from build123d import *

# Parameters (mm, degrees)
EYELID_OUTLINE_R   = 1.25
EYELID_DEPTH       = 3
SKETCH1_R          = 1.5
SKETCH1_W          = 68
SKETCH1_H          = 13
CUT_EXTRUDE1_DEPTH = 48.130138977


# Read off the part's stored shape, not the designer's step: eyelid
with BuildPart() as part:
    # eyelid outline → eyelid (new body)
    with BuildSketch(Plane(origin=(0, 0, 0), x_dir=(1, 0, 0), z_dir=(0, 1, 0))):
        with BuildLine():
            Line((28, -2), (28, -3.803847577))
            ThreePointArc((28, -3.803847577), (27.598076211, -5.303847577), (26.5, -6.401923789))
            ThreePointArc((26.5, -6.401923789), (25.102222521, -9.776457136), (28, -12))
            Line((28, -12), (29.1, -12))
            Line((29.1, -12), (29.1, -16))
            Line((29.1, -16), (30.9, -25))
            Line((30.9, -25), (32.4, -25))
            Line((32.4, -25), (33.9, -23.5))
            Line((33.9, -23.5), (33.9, -22.5))
            Line((33.9, -22.5), (33.4, -22))
            Line((33.4, -22), (32.9, -21))
            Line((32.9, -21), (32.9, -12))
            Line((32.9, -12), (34, -12))
            Line((34, -12), (34, -1.200719678))
            Line((34, -1.200719678), (31.366635055, 8.507890769))
            ThreePointArc((31.366635055, 8.507890769), (0, 32.5), (-31.366635055, 8.507890769))
            Line((-31.366635055, 8.507890769), (-34, -1.200719678))
            Line((-34, -1.200719678), (-34, -12))
            Line((-34, -12), (-32.9, -12))
            Line((-32.9, -12), (-32.9, -21))
            Line((-32.9, -21), (-33.4, -22))
            Line((-33.4, -22), (-33.9, -22.5))
            Line((-33.9, -22.5), (-33.9, -23.5))
            Line((-33.9, -23.5), (-32.4, -25))
            Line((-32.4, -25), (-30.9, -25))
            Line((-30.9, -25), (-29.1, -16))
            Line((-29.1, -16), (-29.1, -12))
            Line((-29.1, -12), (-28, -12))
            ThreePointArc((-28, -12), (-25.102222521, -9.776457136), (-26.5, -6.401923789))
            ThreePointArc((-26.5, -6.401923789), (-27.598076211, -5.303847577), (-28, -3.803847577))
            Line((-28, -3.803847577), (-28, -2))
            Line((-28, -2), (-25.57587166, 6.937203242))
            ThreePointArc((-25.57587166, 6.937203242), (0, 26.5), (25.57587166, 6.937203242))
            Line((25.57587166, 6.937203242), (28, -2))
        make_face()
        with Locations((-28, -9)):
            Circle(EYELID_OUTLINE_R, mode=Mode.SUBTRACT)
        with Locations((28, -9)):
            Circle(EYELID_OUTLINE_R, mode=Mode.SUBTRACT)
    extrude(amount=EYELID_DEPTH)

    # Sketch1 → Cut-Extrude1 (cut, through all)
    with BuildSketch(Plane(origin=(0, 0, 0), x_dir=(1, 0, 0), z_dir=(0, 1, 0))):
        with Locations(Location((-28, -9, 0), (0, 0, 270))):
            Circle(SKETCH1_R)
        with Locations(Location((28, -9, 0), (0, 0, 270))):
            Circle(SKETCH1_R)
        with Locations((0, -18.5)):
            Rectangle(SKETCH1_W, SKETCH1_H)
    extrude(amount=CUT_EXTRUDE1_DEPTH, mode=Mode.SUBTRACT)


solid = part.part
Can you work these out from the model? Positions are in its coordinate system, mm. A direction names the side the tool comes from. Round coordinates to 2 decimals unless told otherwise and drop trailing zeros. Loops run counter-clockwise (first coordinate to the right, second up) from the corner with the lowest first, then second, coordinate; pieces in that order, holes last. Notation, with made-up numbers: (82.5, 43) - (117.5, 43) arc R22 cw to (117.5, 72) - close; hole circle Ø11 at (54.5, 54.5). An arc over 180 degrees is marked (long way). Answer in a Markdown table with one row per item. Add a question column.
Q1. I need wall thicknesses on L1, parallel to X at y = 1, z = 9; L2, parallel to Z at x = 0.5, y = 2.1; L3, parallel to X at y = 0.6, z = -12. Which ranges of each line are inside material? Lowest first, please.
Q2. Which directions (+Z, -Z, +X, -X, +Y, -Y) give clear straight access to the entire face, cutting with the end or side of a thin tool? Please do faces 1 (the flat face through (26.77, 1.48, -2.53)), 2 (the flat face through (32.7, 1.48, -3.59)).
Q3. I want a section at D-D on x = 14. List the corners of the cut face in (y, z) for me, and give its area (3 significant figures).
Q4. I want a section at A-A on y = 1.5. List the corners of the cut face in (x, z) for me, and give its area (3 significant figures).
Q5. We'd pull the mould along Z, two halves only. Please class faces 3 (the flat face through (-26.805, 1.479, -2.406)), 4 (the flat face through (34, 1, 7)), 5 (the flat face through (28, 1, 3)), 6 (the cylindrical face through (0.594, 1.479, -32.495)): pulls with the +Z half, pulls with the -Z half, needs draft (parallel to the pull), parting line crosses it, or undercut.
Q6. I want a section at B-B on z = 9. List the corners of the cut face in (x, y) for me, and give its area (3 significant figures).
Q7. For pin 1 Ø1 at (x, y) = (15, 2) entering from +Z; pin 2 Ø12 at (x, z) = (-19.5, -3.5) entering from -Y, each with a flat end and sliding along its axis, tell me the tip position at first contact or that it passes through.
Q8. I want a section at C-C on z = 0. List the corners of the cut face in (x, y) for me.
A:
| question | item | result |
|---|---|---|
| 1 | L1 | -34 to -29.5, -26.5 to -25, 25 to 26.5, 29.5 to 34 |
| 1 | L2 | -32.5 to -26.5 |
| 1 | L3 | -30.2 to -23.63, 23.63 to 30.2 |
| 2 | face 1 | +Y, -Y |
| 2 | face 2 | -Z, +X, +Y, -Y |
| 3 | outline | (0, -29.33) - (3, -29.33) - (3, -22.5) - (0, -22.5) - close |
| 3 | area | 20.5 mm^2 |
| 4 | outline | (-34, 1.2) - (-31.37, -8.51) arc R32.5 ccw to (31.37, -8.51) - (34, 1.2) - (34, 12) - (28, 12) arc R3 ccw to (26.5, 6.4) arc R3 cw to (28, 3.8) - (28, 2) - (25.58, -6.94) arc R26.5 cw to (-25.58, -6.94) - (-28, 2) - (-28, 3.8) arc R3 cw to (-26.5, 6.4) arc R3 ccw to (-28, 12) - (-34, 12) - close; hole circle Ø3 at (-28, 9); hole circle Ø3 at (28, 9) |
| 4 | area | 719 mm^2 |
| 5 | face 3 | undercut |
| 5 | face 4 | needs draft |
| 5 | face 5 | undercut |
| 5 | face 6 | pulls with the -Z half |
| 6 | outline | (-34, 0) - (-29.5, 0) - (-29.5, 3) - (-34, 3) - close; (-26.5, 0) - (-25, 0) - (-25, 3) - (-26.5, 3) - close; (25, 0) - (26.5, 0) - (26.5, 3) - (25, 3) - close; (29.5, 0) - (34, 0) - (34, 3) - (29.5, 3) - close |
| 6 | area | 36.0 mm^2 |
| 7 | pin 1 | z = -21.49 |
| 7 | pin 2 | through |
| 8 | outline | (-33.67, 0) - (-27.46, 0) - (-27.46, 3) - (-33.67, 3) - close; (27.46, 0) - (33.67, 0) - (33.67, 3) - (27.46, 3) - close |
